For this review, take the finished solid that the model builds, in its own axes (mm). Face numbers are marked on the shaded views. A direction names the side the tool comes from. Give positions to 0.01 mm unless a question says otherwise; leave off trailing zeros. Order: outer loops, then holes, each group sorted by start corner. A loop starts at its lowest first (then second) coordinate and runs counter-clockwise, first axis right, second up. Notation, with made-up numbers: (29, 10) - (82, 10) arc R18 ccw to (82, 32) - close; hole circle Ø10 at (-5.75, 22). An arc over 180 degrees is marked (long way). Answer as a JSON object with one key per item and string values. Group by question number.
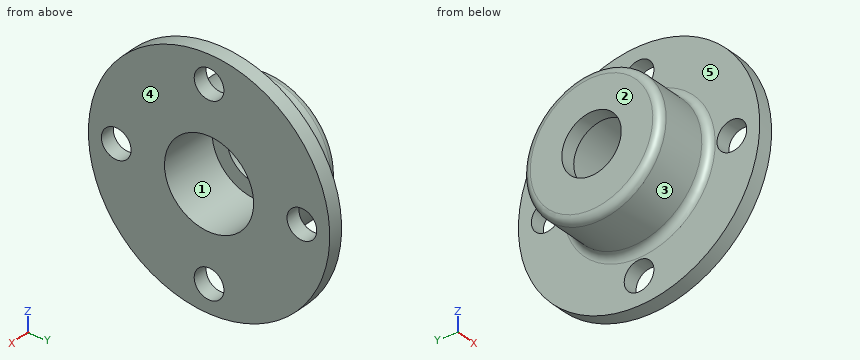
from build123d import *

# Parameters (mm, degrees)
SKETCH5_R          = 25.4
CUT_EXTRUDE1_DEPTH = 310.07425534
CIRPATTERN1_COUNT  = 4
FILLET1_R          = 12.7


with BuildPart() as part:
    # Sketch1 → Revolve6 (revolve)
    with BuildSketch(Plane(origin=(0, 0, 0), x_dir=(1, 0, 0), z_dir=(0, 1, 0)), mode=Mode.PRIVATE) as revolve6_sk:
        Polygon((0, 50.8), (0, 117.502925505), (101.6, 117.502925505), (101.6, 206.402925505), (127, 206.402925505), (127, 76.2), (25.4, 76.2), (25.4, 50.8), align=None)
    revolve(revolve6_sk.sketch.rotate(Axis((-155.979583507, 0, 0), (1, 0, 0)), 180), axis=Axis((-155.979583507, 0, 0), (1, 0, 0)))

    # Sketch5 → Cut-Extrude1 (cut, through all)
    with BuildSketch(Plane.ZY.offset(-101.6)):
        with Locations((0, 158.75)):
            Circle(SKETCH5_R)
    cut_extrude1 = extrude(amount=-CUT_EXTRUDE1_DEPTH, mode=Mode.SUBTRACT)

    # CirPattern1: Cut-Extrude1 ×4 about axis
    cirpattern1_axis = Axis((0, 0, 0), (1, 0, 0))
    for i in range(1, CIRPATTERN1_COUNT):
        add(cut_extrude1.rotate(cirpattern1_axis, i * 360 / CIRPATTERN1_COUNT), mode=Mode.SUBTRACT)

    # Fillet1
    fillet1_edges = [part.edges().sort_by_distance(p)[0] for p in [
        (0, 0, -117.502925505),
        (101.6, 0, -117.502925505),
    ]]
    fillet(fillet1_edges, radius=FILLET1_R)


solid = part.part
1) Consider section B-B (y = 171). Give the boundary of the cut face in (x, z), plus the area to 3 significant figures.
2) For pin 1 (8 mm diameter, centred on x = 75.5, z = 83, fed in from +Y); pin 2 (10 mm diameter, centred on x = 57, y = 32.5, fed in from -Z); pin 3 (4 mm diameter, centred on x = 108.5, z = -28.5, fed in from +Y), all flat-tipped, find the tip position at first contact; note any pin that passes through.
3) For the marked faces 4 and 5, list the 3-axis set-ups (+Z, -Z, +X, -X, +Y, -Y) from which the entire face can be reached by the end or side of a thin tool; tool diameter is ignored.
4) Mouldability with a two-part tool opening along Y and no side actions: class the marked faces 1, 2 and 3 as released by +Y, released by -Y, zero draft, split by the parting line, or undercut.
5) Consider section C-C (x = 49). Give the boundary of the cut face in (y, z).
6) For line 1 (X direction, y = -159, z = -90.5); line 2 (Y direction, x = 107, z = 13); line 3 (Z direction, x = 80.5, y = 18), list the stretches that pass through material, from the lowest coordinate up.
7) Consider section D-D (z = 174.5). Give the boundary of the cut face in (x, y), plus the area to 3 significant figures.
8) Consider section A-A (y = 0). Give the boundary of the cut face in (x, z).
Result set:
{
 "1": {"outline": "(101.6, -115.59) - (127, -115.59) - (127, -22.25) - (101.6, -22.25) - close; (101.6, 22.25) - (127, 22.25) - (127, 115.59) - (101.6, 115.59) - close", "area": "4,740 mm2"},
 "2": {"pin 1": "stops at y = 86.98", "pin 2": "stops at z = -114.24", "pin 3": "stops at y = 204.69"},
 "3": {"face 4": "+Z, -Z, +X, +Y, -Y", "face 5": "-X"},
 "4": {"face 1": "undercut", "face 2": "zero draft", "face 3": "split by the parting line"},
 "5": {"outline": "circle Ø235.01 at (0, 0); hole circle Ø152.4 at (0, 0)"},
 "6": {"line 1": "x = 101.6 to 127", "line 2": "y = -205.99 to -180.57, -136.93 to -75.08, 75.08 to 136.93, 180.57 to 205.99", "line 3": "z = -116.12 to -74.04, 74.04 to 116.12"},
 "7": {"outline": "(101.6, -110.24) - (127, -110.24) - (127, -19.93) - (101.6, -19.93) - close; (101.6, 19.93) - (127, 19.93) - (127, 110.24) - (101.6, 110.24) - close", "area": "4,590 mm2"},
 "8": {"outline": "(0, -104.8) arc R12.7 ccw to (12.7, -117.5) - (88.9, -117.5) arc R12.7 cw to (101.6, -130.2) - (101.6, -133.35) - (127, -133.35) - (127, -76.2) - (25.4, -76.2) - (25.4, -50.8) - (0, -50.8) - close; (0, 50.8) - (25.4, 50.8) - (25.4, 76.2) - (127, 76.2) - (127, 133.35) - (101.6, 133.35) - (101.6, 130.2) arc R12.7 cw to (88.9, 117.5) - (12.7, 117.5) arc R12.7 ccw to (0, 104.8) - close; (101.6, -206.4) - (127, -206.4) - (127, -184.15) - (101.6, -184.15) - close; (101.6, 184.15) - (127, 184.15) - (127, 206.4) - (101.6, 206.4) - close"}
}
